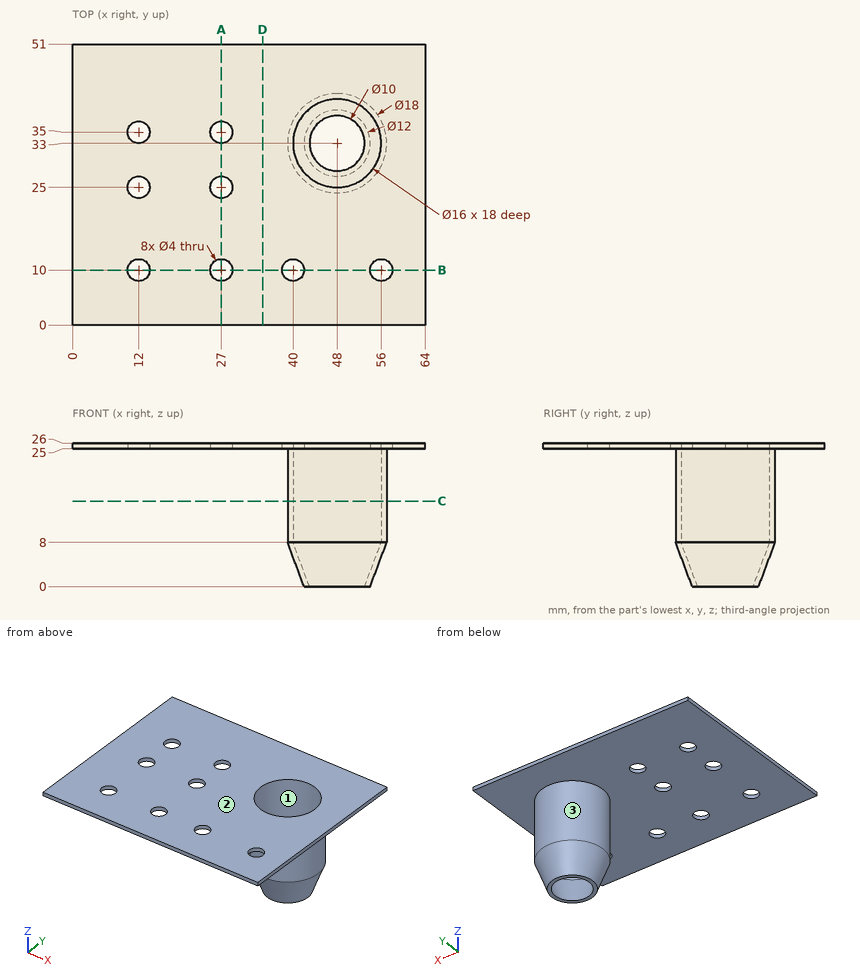
Geometry: see drawing. Coordinates: mm, zero at the bounding-box minimum. Round coordinates to 2 decimals unless told otherwise and drop trailing zeros. Write each loop counter-clockwise with the first axis right and the second up, starting at its lowest first coordinate (ties: lowest second). Pieces come first, ordered by that corner, then holes. Notation, with made-up numbers: M 6.5,1.25 L 64.5,1.25 A27 ccw 64.5,31.25 Z; hole C -33,77.5 d2. An arc over 180 degrees is marked long. Answer in a Markdown table with one row per item. Add a question column.
(1) Contact query for flat-ended pins moving along their axis: pin 1 (6 mm diameter, centred on x = 46.5, z = 5, fed in from -Y); pin 2 (4 mm diameter, centred on y = 32, z = 8, fed in from -X); pin 3 (4.5 mm diameter, centred on x = 12, y = 10, fed in from -Z); pin 4 (2.5 mm diameter, centred on x = 12, y = 35, fed in from +Z). Output: stop coordinate, or through.
(2) Ray query, L1, parallel to Y at x = 12, z = 25.4; L2, parallel to X at y = 35, z = 25.45; L3, parallel to Z at x = 42.5, y = 43.5. Return the intervals inside material, ascending.
(3) Cut plane B-B, the plane y = 10. Return the cut outline in (x, z).
(4) Cut plane A-A, the plane x = 27. Return the cut outline in (y, z).
(5) Cut plane D-D, the plane x = 34.5. Return the cut outline in (y, z).
(6) Cut plane C-C, the plane z = 15.5. Return the cut outline in (x, y), then the cut area to 3 significant figures.
(7) Draft query along X for the marked faces 1, 2 and 3. Return one class per face: pulls with the +X half, pulls with the -X half, needs draft (parallel to the pull), parting line crosses it, or undercut.
Established:
| question | item | result |
|---|---|---|
| 1 | pin 1 | y = 24.07 |
| 1 | pin 2 | x = 39 |
| 1 | pin 3 | z = 25 |
| 1 | pin 4 | through |
| 2 | L1 | 0 to 8, 12 to 23, 27 to 33, 37 to 51 |
| 2 | L2 | 0 to 10, 14 to 25, 29 to 40.25, 55.75 to 64 |
| 2 | L3 | 25 to 26 |
| 3 | outline | M 0,25 L 10,25 L 10,26 L 0,26 Z; M 14,25 L 25,25 L 25,26 L 14,26 Z; M 29,25 L 38,25 L 38,26 L 29,26 Z; M 42,25 L 54,25 L 54,26 L 42,26 Z; M 58,25 L 64,25 L 64,26 L 58,26 Z |
| 4 | outline | M 0,25 L 8,25 L 8,26 L 0,26 Z; M 12,25 L 23,25 L 23,26 L 12,26 Z; M 27,25 L 33,25 L 33,26 L 27,26 Z; M 37,25 L 51,25 L 51,26 L 37,26 Z |
| 5 | outline | M 0,25 L 51,25 L 51,26 L 0,26 Z |
| 6 | outline | C 48,33 d18; hole C 48,33 d16 |
| 6 | area | 53.4 mm² |
| 7 | face 1 | undercut |
| 7 | face 2 | needs draft |
| 7 | face 3 | parting line crosses it |
